Autodesk Inventor part; units mm, degrees
ref_plane "YZ Plane" through (0, 0, 0) normal (1, 0, 0) x (0, 1, 0)
ref_plane "XZ Plane" through (0, 0, 0) normal (0, 1, 0) x (-1, 0, 0)
ref_plane "XY Plane" through (0, 0, 0) normal (0, 0, 1) x (1, 0, 0)
sketch "Boceto1" plane through (0, 0, 0) normal (0, 1, 0) x (-1, 0, 0)
  line L0 (-25, 60) -> (25, 60)
  line L1 (25, 60) -> (25, -60)
  line L2 (25, -60) -> (-25, -60)
  line L3 (-25, -60) -> (-25, 60)
  line L4 (-25, 60) -> (25, -60) construction
  line L5 (25, 60) -> (-25, -60) construction
  circle A0 centre (19, 50) radius 2.7
  circle A1 centre (-19, 50) radius 2.7
  circle A2 centre (19, -50) radius 2.7
  circle A3 centre (-19, -50) radius 2.7
  point P0 (0, 0)
  dimension "d0" = 120
  dimension "d1" = 50
  dimension "d2" = 5.4
  dimension "d3" = 6
  dimension "d4" = 6
  dimension "d5" = 10
  dimension "d6" = 10
  dimension "d7" = 10
extrude "Extrusión1" add sketch "Boceto1" along normal blind 35
sketch "Boceto2" plane through (-25, 0, -60) normal (-1, 0, 0) x (0, 0, 1)
  circle A0 centre (60, 8) radius 3
  line L0 (0, 0) -> (120, 0)
  line L1 (120, 0) -> (0, 0)
  point P0 (60, 0)
  point P1 (60, 0)
  dimension "d10" = 6
  dimension "d11" = 8
extrude "Extrusión2" cut sketch "Boceto2" against normal through all
sketch "Boceto3" plane through (25, 0, 60) normal (1, 0, 0) x (0, 0, -1)
  circle A0 centre (60, 42.6) radius 12.5
  line L0 (0, 35) -> (120, 35)
  line L1 (0, 0) -> (120, 0)
  point P0 (60, 0)
  point P1 (60, 0)
  dimension "d14" = 25
  dimension "d15" = 7.6
extrude "Extrusión3" cut sketch "Boceto3" against normal through all
sketch "Boceto4" plane through (25, 0, 60) normal (1, 0, 0) x (0, 0, -1)
  circle A0 centre (60, 42.6) radius 18
  point P0 (60, 0)
extrude "Extrusión4" cut sketch "Boceto4" against normal blind 104.5
sketch "Boceto5" plane through (25, 0, 60) normal (1, 0, 0) x (0, 0, -1)
  arc A0 (43.6831, 35) -> (76.3169, 35) centre (60, 42.6) ccw
  circle A1 centre (60, 42.6) radius 19
  point P0 (60, 0)
  dimension "d20" = 1
extrude "Extrusión5" cut sketch "Boceto5" against normal through all
fillet "Empalme1" radius 2 6 edges at (0, 0, 60) (0, 35, 60) (0, 35, -60) (0, 0, -60) (0, 35, -17.4138) (0, 35, 17.4138)
properties part number "LowerSupport"
Could you check a few things on this model? Use its own coordinates, in mm. Round coordinates to 2 decimals unless told otherwise and drop trailing zeros. Loops run counter-clockwise (first coordinate to the right, second up) from the corner with the lowest first, then second, coordinate; pieces in that order, holes last. Notation, with made-up numbers: (8.25, 30) - (18.25, 30) arc R20 cw to (18.25, 60) - close; hole circle Ø10 at (2, 7). An arc over 180 degrees is marked (long way). Answer in a Markdown table with one row per item. Add a question column.
(1) If we section it at D-D (z = 0): Please give me the cut outline in (x, y), plus the area to 3 significant figures.
(2) If we section it at B-B (y = 8): Please give me the cut outline in (x, z), plus the area to 3 significant figures.
(3) If we mould it in two halves opening along X, with no side actions, what happens to faces 1 (the face through (0, 35, -38)), 2 (the face through (25, 17, -1)), 3 (the face through (-20.246, 17.255, -47.605))? For each: pulls with the +X half, pulls with the -X half, needs draft (parallel to the pull), parting line crosses it, or undercut.
(4) If we section it at C-C (z = -50): Please give me the cut outline in (x, y).
(5) I need wall thicknesses on line 1 along Z through (x, y) = (19, 20); line 2 along Z through (x, y) = (20.5, 8.5) (3 decimals); line 3 along Z through (x, y) = (-19, 26). Which ranges of each line are inside material? Lowest first, please.
(6) I'm going to push flat-ended pins straight in: pin 1 (3 mm diameter, centred on x = -7.5, z = -10.5, fed in from +Y); pin 2 (5.5 mm diameter, centred on y = 8, z = 0, fed in from +X). Where does each tip first touch, or does it pass through?
(7) If we section it at A-A (x = -19): Please give me the cut outline in (y, z), plus the area to 3 significant figures.
Model answer:
| question | item | result |
|---|---|---|
| 1 | outline | (-25, 0) - (25, 0) - (25, 5) - (-25, 5) - close; (-25, 11) - (25, 11) - (25, 23.6) - (-25, 23.6) - close |
| 1 | area | 880 mm² |
| 2 | outline | (-25, -60) - (25, -60) - (25, -3) - (-25, -3) - close; (-25, 3) - (25, 3) - (25, 60) - (-25, 60) - close; hole circle Ø5.4 at (-19, -50); hole circle Ø5.4 at (-19, 50); hole circle Ø5.4 at (19, -50); hole circle Ø5.4 at (19, 50) |
| 2 | area | 5,610 mm² |
| 3 | face 1 | needs draft |
| 3 | face 2 | pulls with the +X half |
| 3 | face 3 | undercut |
| 4 | outline | (-25, 0) - (-21.7, 0) - (-21.7, 35) - (-25, 35) - close; (-16.3, 0) - (16.3, 0) - (16.3, 35) - (-16.3, 35) - close; (21.7, 0) - (25, 0) - (25, 35) - (21.7, 35) - close |
| 5 | line 1 | z = -60 to -52.7, -47.3 to 47.3, 52.7 to 60 |
| 5 | line 2 | z = -60 to -52.245, -47.755 to -2.958, 2.958 to 47.755, 52.245 to 60 |
| 5 | line 3 | z = -60 to -52.7, -47.3 to -9.24, 9.24 to 47.3, 52.7 to 60 |
| 6 | pin 1 | stops at y = 27.87 |
| 6 | pin 2 | passes through |
| 7 | outline | (0, -58) arc R2 ccw to (2, -60) - (33, -60) arc R2 ccw to (35, -58) - (35, -52.7) - (0, -52.7) - close; (0, -47.3) - (35, -47.3) - (35, -18.68) arc R2 ccw to (33.91, -16.9) arc R19 cw to (33.91, 16.9) arc R2 ccw to (35, 18.68) - (35, 47.3) - (0, 47.3) - close; (0, 52.7) - (35, 52.7) - (35, 58) arc R2 ccw to (33, 60) - (2, 60) arc R2 ccw to (0, 58) - close; hole circle Ø6 at (8, 0) |
| 7 | area | 3,500 mm² |
